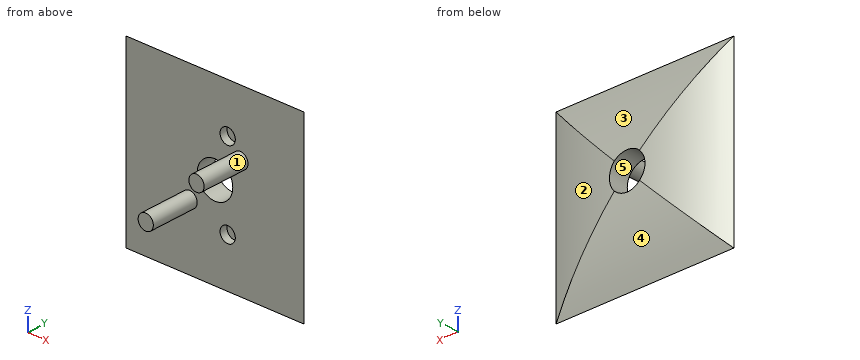
Autodesk Inventor part; units mm, degrees
ref_plane "YZ Plane" through (0, 0, 0) normal (1, 0, 0) x (0, 1, 0)
ref_plane "XZ Plane" through (0, 0, 0) normal (0, 1, 0) x (-1, 0, 0)
ref_plane "XY Plane" through (0, 0, 0) normal (0, 0, 1) x (1, 0, 0)
sketch "Sketch1" plane through (0, 0, 0) normal (0, 1, 0) x (-1, 0, 0)
  line L0 (17.5, -17.5) -> (-17.5, -17.5)
  line L1 (-17.5, -17.5) -> (-17.5, 17.5)
  line L2 (-17.5, 17.5) -> (17.5, 17.5)
  line L3 (17.5, 17.5) -> (17.5, -17.5)
  line L4 (17.5, -17.5) -> (-17.5, 17.5) construction
  line L5 (-17.5, -17.5) -> (17.5, 17.5) construction
  point P0 (0, 0)
  dimension "d0" = 35
  dimension "d1" = 35
extrude "Extrusion1" add sketch "Sketch1" along normal blind 4
sketch "Sketch3" plane through (17.5, 0, 17.5) normal (1, 0, 0) x (0, 0, -1)
  line L0 (35, 4) -> (0, 4)
  line L1 (0, 0) -> (35, 0)
  line L2 (0, 0) -> (35, 0)
  arc A0 (35, 0) -> (0, 0) centre (17.5, -36.2813) ccw
  point P0 (17.5, 4)
extrude "Extrusion3" cut sketch "Sketch3" against normal through all keep common part
sketch "Sketch4" plane through (17.5, 0, -17.5) normal (0, 0, -1) x (-1, 0, 0)
  line L0 (35, 0) -> (35, 4)
  line L1 (0, 0) -> (35, 0)
  line L2 (0, 0) -> (0, 4)
  line L3 (35, 0) -> (0, 0)
  arc A0 (35, 0) -> (0, 0) centre (17.5, -36.2812) ccw
  point P0 (17.5, 0)
  dimension "d31" = 4
extrude "Extrusion4" cut sketch "Sketch4" against normal through all keep common part
sketch "Sketch5" plane through (0, 0, 0) normal (0, -1, 0) x (1, 0, 0)
  circle A0 centre (0, 0) radius 3.5
  dimension "d14" = 7
extrude "Extrusion5" cut sketch "Sketch5" against normal through all
sketch "Sketch6" plane through (0, 0, 0) normal (0, -1, 0) x (1, 0, 0)
  circle A0 centre (-5, -5) radius 1.5
  circle A1 centre (5, 5) radius 1.5
  circle A2 centre (5, -5) radius 1.5
  circle A3 centre (-5, 5) radius 1.5
  point P0 (0, 0)
  point P1 (0, 0)
  dimension "d17" = 3
  dimension "d18" = 3
  dimension "d19" = 5
  dimension "d20" = 5
  dimension "d21" = 5
  dimension "d22" = 5
  dimension "d25" = 3
  dimension "d26" = 3
  dimension "d27" = 5
  dimension "d28" = 5
  dimension "d29" = 5
  dimension "d30" = 5
extrude "Extrusion6" add sketch "Sketch6" along normal blind 9.5 contours A0 | A1
sketch "Sketch7" plane through (0, 0, 0) normal (0, -1, 0) x (1, 0, 0)
  line L0 (-17.5, 17.5) -> (-17.5, -17.5) construction
  line L1 (-17.5, 0) -> (17.5, 0) construction
  line L2 (17.5, -17.5) -> (17.5, 17.5) construction
  circle A0 centre (2.5, 8.124) radius 1.5
  circle A1 centre (2.5, -8.124) radius 1.5
  point P0 (0, 0)
  dimension "d32" = 3
  dimension "d33" = 8.5
  dimension "d34" = 15
extrude "Extrusion7" cut sketch "Sketch7" against normal blind 1.5
equation "\"d1\" = d0"
equation "\"d17\" = d18"
equation "\"d25\" = d18"
equation "\"d26\" = d18"
properties part number "thumper-bumper-trigger-v2"
Part model, mm, in its own coordinate system. Face numbers are marked on the shaded views. A direction names the side the tool comes from. Coordinates: 2 decimals unless noted, no trailing zeros. Order: outer loops, then holes, each group sorted by start corner. A loop starts at its lowest first (then second) coordinate and runs counter-clockwise, first axis right, second up. Notation, with made-up numbers: (61, 14) -> (91, 14) arc R6 cw to (91, 20) -> close; hole circle Ø5 at (19, 62.25). An arc over 180 degrees is marked (long way). Put each result on its own line as item: value. Start each with the question number.
(1) Mould opens along Z. For the marked faces 3, 4 and 5 say: pulls with the +Z half, pulls with the -Z half, needs draft (parallel to the pull), parting line crosses it, or undercut.
(2) Probe line 1 along Z through (x, y) = (2.5, 1.05); line 2 along Z through (x, y) = (2.5, 0.3); line 3 along X through (y, z) = (0.5, 9.5). List the from-to ranges inside material, lowest first. Write a range as [from, to].
(3) Pin check, flat tips, straight feed: pin 1 Ø6.5 at (x, z) = (0, 0) entering from -Y; pin 2 Ø6 at (x, z) = (11.5, 5.5) entering from +Y; pin 3 Ø1.5 at (x, z) = (2, 7.5) entering from -Y; pin 4 Ø8 at (y, z) = (1.5, 13) entering from -X. Stop position of each tip, or through.
(4) Band-saw the part on B-B (z = 0). Give the cut face in (x, y).
(5) Band-saw the part on D-D (y = -3.25). Give the cut face in (x, z), then the cut area to 3 significant figures.
(6) Which spindle directions (+Z, -Z, +X, -X, +Y, -Y) get a long thin tool onto all of the face, cutting with end or side? Do the marked faces 1 and 2. Say none if no direction does.
(7) Band-saw the part on A-A (x = 0). Give the cut face in (y, z), then the cut area to 3 significant figures.
(8) Band-saw the part on C-C (y = 0.5). Give the cut face in (x, z).
Determined:
1. face 3: pulls with the +Z half
1. face 4: pulls with the -Z half
1. face 5: undercut
2. line 1: z = [-15.13, -9.62], [-6.62, -2.45], [2.45, 6.62], [9.62, 15.13]
2. line 2: z = [-16.86, -9.62], [-6.62, -2.45], [2.45, 6.62], [9.62, 16.86]
2. line 3: x = [-16.42, 1.9], [3.1, 16.42]
3. pin 1: passes through
3. pin 2: stops at y = 3.09
3. pin 3: stops at y = 0
3. pin 4: stops at x = -17.5
4. outline: (-17.5, 0) -> (-3.5, 0) -> (-3.5, 3.85) arc R40.28 ccw to start; (3.5, 0) -> (17.5, 0) arc R40.28 ccw to (3.5, 3.85) -> close
5. outline: circle Ø3 at (-5, -5); circle Ø3 at (5, 5)
5. area: 14.1 mm²
6. face 1: -Y
6. face 2: +Z, -Z, +X, +Y
7. outline: (0, -17.5) arc R40.28 ccw to (3.85, -3.5) -> (0, -3.5) -> close; (0, 3.5) -> (3.85, 3.5) arc R40.28 ccw to (0, 17.5) -> close
7. area: 66.7 mm²
8. outline: (-16.42, -16.42) -> (16.42, -16.42) -> (16.42, 16.42) -> (-16.42, 16.42) -> close; hole circle Ø7 at (0, 0); hole circle Ø3 at (2.5, -8.12); hole circle Ø3 at (2.5, 8.12)
